Could you check a few things on this model? Use its own coordinates, in mm. A direction names the side the tool comes from. Give positions to 0.01 mm unless a question says otherwise; leave off trailing zeros. Write each loop counter-clockwise with the first axis right and the second up, starting at its lowest first coordinate (ties: lowest second). Pieces come first, ordered by that corner, then holes. Notation, with made-up numbers: M 0,-18.75 L 24,-18.75 A19 cw 24,-0.75 Z; hole C 35,-7 d9. An arc over 180 degrees is marked long. Use one line per item in the form item = value.
Autodesk Fusion 360 part; units mm, degrees
sketch "Sketch1" plane through (0, 0, 0) normal (0, 0, 1) x (1, 0, 0)
  line L0 (20, -12.5) -> (-20, -12.5)
  line L1 (-20, -12.5) -> (-20, 12.5)
  line L2 (-20, 12.5) -> (20, 12.5)
  line L3 (20, 12.5) -> (20, -12.5)
  line L4 (20, -12.5) -> (-20, 12.5) construction
  line L5 (-20, -12.5) -> (20, 12.5) construction
  dimension "d1" = 40
  dimension "d2" = 25
extrude "Extrude1" add sketch "Sketch1" along normal blind 12.7
sketch "Sketch2" plane through (0, 0, 12.7) normal (0, 0, 1) x (-1, 0, 0)
  line L0 (-20, -12.5) -> (20, -12.5)
  line L1 (20, -12.5) -> (20, 12.5)
  line L2 (20, 12.5) -> (-20, 12.5)
  line L3 (-20, 12.5) -> (-20, -12.5)
  line L4 (-20, 7.5) -> (20, 7.5)
  line L5 (20, 7.5) -> (20, -7.5)
  line L6 (20, -7.5) -> (-20, -7.5)
  line L7 (-20, -7.5) -> (-20, 7.5)
  line L8 (-20, 7.5) -> (20, -7.5) construction
  line L9 (20, 7.5) -> (-20, -7.5) construction
  dimension "d5" = 40
  dimension "d6" = 15
extrude "Extrude2" cut sketch "Sketch2" against normal blind 2 contours L1 L3 L4 L5 L6 L7
sketch "Sketch3" plane through (0, -12.5, 0) normal (0, -1, 0) x (1, 0, 0)
  line L0 (-20, 0) -> (20, 0)
  line L1 (20, 0) -> (20, 12.7)
  line L2 (20, 12.7) -> (-20, 12.7)
  line L3 (-20, 12.7) -> (-20, 0)
  line L4 (0, 12.7) -> (0, 0) construction
  line L5 (20, 0) -> (10, 0)
  line L6 (10, 0) -> (10, 3)
  line L7 (10, 3) -> (20, 3)
  line L8 (20, 3) -> (20, 0)
  line L9 (-20, 0) -> (-10, 0)
  line L10 (-10, 0) -> (-10, 3)
  line L11 (-10, 3) -> (-20, 3)
  line L12 (-20, 3) -> (-20, 0)
  point P0 (0, 12.7)
  dimension "d23" = 10
  dimension "d24" = 3
  dimension "d25" = 10
  dimension "d26" = 3
extrude "Extrude5" add sketch "Sketch3" along normal blind 20 contours L0 L3 L9 L10 L11 L12 | L0 L1 L5 L6 L7 L8
sketch "Sketch6" plane through (0, 12.5, 0) normal (0, 1, 0) x (-1, 0, 0)
  line L0 (-20, 0) -> (20, 0)
  line L1 (20, 0) -> (20, 12.7)
  line L2 (20, 12.7) -> (-20, 12.7)
  line L3 (-20, 12.7) -> (-20, 0)
  line L4 (-10, 3) -> (-20, 3)
  line L5 (-10, 0) -> (-10, 3)
  line L6 (-20, 0) -> (-10, 0)
  line L7 (-20, 3) -> (-20, 0)
  line L8 (10, 0) -> (10, 3)
  line L9 (10, 3) -> (20, 3)
  line L10 (20, 0) -> (10, 0)
  line L11 (20, 3) -> (20, 0)
  line L12 (-20, 0) -> (-10, 0)
  line L13 (-10, 0) -> (-10, 3)
  line L14 (-10, 3) -> (-20, 3)
  line L15 (-20, 3) -> (-20, 0)
  line L16 (20, 0) -> (10, 0)
  line L17 (10, 0) -> (10, 3)
  line L18 (10, 3) -> (20, 3)
  line L19 (20, 3) -> (20, 0)
extrude "Extrude6" add sketch "Sketch6" along normal blind 20 contours L0 L3 L4 L5 L6 L7 L12 L13 L14 L15 | L0 L1 L8 L9 L10 L11 L16 L17 L18 L19
fillet "Fillet5" radius 2 10 edges at (-10, 12.5, 1.5) (-15, 12.5, 3) (15, 12.5, 3) (0, 12.5, 12.7) (0, -12.5, 12.7) (10, 12.5, 1.5) (-15, -12.5, 3) (10, -12.5, 1.5) (15, -12.5, 3) (-10, -12.5, 1.5)
fillet "Fillet6" radius 5 8 edges at (-20, -32.5, 1.5) (-10, -32.5, 1.5) (10, -32.5, 1.5) (20, -32.5, 1.5) (-10, 32.5, 1.5) (20, 32.5, 1.5) (-20, 32.5, 1.5) (10, 32.5, 1.5)
equation "d3 = 25.4 mm / 2"
equation "d25 = d23"
equation "d26 = d24"
1) For pin 1 Ø0.6 at (x, z) = (0, 11.5) entering from -Y; pin 2 Ø1 at (x, z) = (-3.5, 12) entering from +Y; pin 3 Ø11 at (x, y) = (17, 24) entering from +Z, each with a flat end and sliding along its axis, tell me the tip position at first contact or that it passes through.
Checked values:
pin_1 = -12.44
pin_2 = 12.33
pin_3 = 3
2) I want a section at D-D, the plane y = 5. Please give me the cut outline in (x, z).
Checked values:
outline = M -20,0 L 20,0 L 20,10.7 L -20,10.7 Z
3) Thinking about a two-plate mould opening in Y: for faces 1 (the flat face through (0, -7.5, 12)), 2 (the cylindrical face through (9.43, -13.1, 1.98)), 3 (the flat face through (0, 0, 0)), which applies, released by +Y, released by -Y, zero draft, split by the parting line, or undercut?
Checked values:
face_1 = undercut
face_2 = released by -Y
face_3 = zero draft
4) For faces 4 (the cylindrical face through (11.43, -31, 1.52)), 5 (the flat face through (-15, 23, 3)), 6 (the flat face through (10, 21, 1)), which set-ups out of +Z, -Z, +X, -X, +Y, -Y let a thin tool reach every point of the face, with its end or its side?
Checked values:
face_4 = +Z, -Z, -Y
face_5 = +Z, +X, -X, +Y
face_6 = +Z, -Z, +Y
5) If I drill on L1, parallel to X at y = -22, z = 2.5; L2, parallel to Y at x = -15.5, z = 6; L3, parallel to Z at x = -6, y = -1, over which ranges is the centre line in solid material (lowest first)?
Checked values:
L1 = -20 to -10, 10 to 20
L2 = -12.5 to 12.5
L3 = 0 to 10.7
6) I want a section at B-B, the plane x = -3.5. Please give me the cut outline in (y, z), plus the area to 3 significant figures.
Checked values:
outline = M -12.5,0 L 12.5,0 L 12.5,10.7 A2 ccw 10.5,12.7 L 7.5,12.7 L 7.5,10.7 L -7.5,10.7 L -7.5,12.7 L -10.5,12.7 A2 ccw -12.5,10.7 Z
area = 286 mm2
7) I want a section at A-A, the plane y = 18.5. Please give me the cut outline in (x, z).
Checked values:
outline = M -20,0 L -10,0 L -10,3 L -20,3 Z; M 10,0 L 20,0 L 20,3 L 10,3 Z
8) I want a section at C-C, the plane z = 8.75. Please give me the cut outline in (x, y), plus the area to 3 significant figures.
Checked values:
outline = M -20,-12.5 L 20,-12.5 L 20,12.5 L -20,12.5 Z
area = 1,000 mm2
